from build123d import *

# Parameters (mm, degrees)
F1_DEPTH = 20
F0_R     = 12.5
F2_DEPTH = 20


# Not quite as in the source:
# - a feature names something its author has since deleted; it is built from what else it names


with BuildPart() as f1:
    # F0 (on Front) → F1 (new body)
    with BuildSketch(Plane.XZ):
        with BuildLine():
            Line((-0.6229226271, -45), (-0.6229226271, 45))
            Line((-0.6229226271, 45), (-76.0821841814, 29.3769813899))
            ThreePointArc((-76.0821841814, 29.3769813899), (-51.0588480477, 23.2644097866), (-40, 0))
            ThreePointArc((-40, 0), (-51.0588480477, -23.2644097866), (-76.0821841814, -29.3769813899))
            Line((-76.0821841814, -29.3769813899), (-0.6229226271, -45))
        make_face()
    extrude(amount=F1_DEPTH)

    # F0 (on Front) → F2 (join)
    with BuildSketch(Plane.XZ):
        with BuildLine():
            ThreePointArc((-40, 0), (-51.0588480477, 23.2644097866), (-76.0821841814, 29.3769813899))
            ThreePointArc((-76.0821841814, 29.3769813899), (-100, 0), (-76.0821841814, -29.3769813899))
            ThreePointArc((-76.0821841814, -29.3769813899), (-51.0588480477, -23.2644097866), (-40, 0))
        make_face()
        with Locations((-70, 0)):
            Circle(F0_R, mode=Mode.SUBTRACT)
    extrude(amount=F2_DEPTH)


solid = f1.part
The listing builds one solid part. Answer for the finished solid, in the listing's coordinates (mm). Round coordinates to 2 decimals unless told otherwise and drop trailing zeros. Write each loop counter-clockwise with the first axis right and the second up, starting at its lowest first coordinate (ties: lowest second). Pieces come first, ordered by that corner, then holes. Notation, with made-up numbers: (-5.5, 8.5) - (23.5, 8.5) arc R23 ccw to (23.5, 47.5) - close; hole circle Ø10 at (-31.5, 83). An arc over 180 degrees is marked (long way). Use one line per item in the form item = value. Start each with the question number.
Item 1: Flat-ended cylindrical pins translate along their axes: pin 1 Ø3 at (x, z) = (-60.5, 2) entering from +Y; pin 2 Ø4 at (x, y) = (-90, -14.5) entering from +Z; pin 3 Ø12 at (x, y) = (-81.5, -10) entering from -Z; pin 4 Ø8 at (x, y) = (-33, -10) entering from +Z. Find the tip coordinate at first contact, or state that the pin passes through.
Item 2: A cutting plane is placed at A-A (z = 0). Write down the section's boundary in (x, y), plus the area to 3 significant figures.
Item 3: A cutting plane is placed at D-D (z = 24). Write down the section's boundary in (x, y), plus the area to 3 significant figures.
Item 4: Determine the mould class of faces 1 (the cylindrical face through (-82.488, -9.86, 0.55)), 2 (the flat face through (-38.88, -9.86, -37.08)), 3 (the flat face through (-0.623, -10, -1)) for opening direction Z: +Z half, -Z half, draft (parallel to the pull), parting line (faces both ways), or undercut.
Item 5: A cutting plane is placed at C-C (y = -8.5). Write down the section's boundary in (x, z), plus the area to 3 significant figures.
Item 6: Find the intervals of material crossed by line 1 (Z direction, x = -70, y = -12.25); line 2 (Z direction, x = -81, y = -15); line 3 (X direction, y = -16.25, z = -5.5), in increasing order. Write a range as [from, to].
Item 7: A cutting plane is placed at B-B (x = -70). Write down the section's boundary in (y, z).
The answers:
q1.pin_1 = through
q1.pin_2 = 24
q1.pin_3 = -29.5
q1.pin_4 = 39.12
q2.outline = (-100, -20) - (-82.5, -20) - (-82.5, 0) - (-100, 0) - close; (-57.5, -20) - (-0.62, -20) - (-0.62, 0) - (-57.5, 0) - close
q2.area = 1,490 mm^2
q3.outline = (-88, -20) - (-0.62, -20) - (-0.62, 0) - (-88, 0) - close
q3.area = 1,750 mm^2
q4.face_1 = undercut
q4.face_2 = -Z half
q4.face_3 = draft
q5.outline = (-76.08, -29.38) - (-0.62, -45) - (-0.62, 45) - (-76.08, 29.38) arc R30 ccw to start; hole circle Ø25 at (-70, 0)
q5.area = 6,170 mm^2
q6.line_1 = [-30.64, -12.5], [12.5, 30.64]
q6.line_2 = [-27.91, -5.94], [5.94, 27.91]
q6.line_3 = [-99.49, -81.22], [-58.78, -0.62]
q7.outline = (-20, -30.64) - (0, -30.64) - (0, -12.5) - (-20, -12.5) - close; (-20, 12.5) - (0, 12.5) - (0, 30.64) - (-20, 30.64) - close
